The listing builds one solid part. Answer for the finished solid, in the listing's coordinates (mm). Round coordinates to 2 decimals unless told otherwise and drop trailing zeros. Loops run counter-clockwise (first coordinate to the right, second up) from the corner with the lowest first, then second, coordinate; pieces in that order, holes last. Notation, with made-up numbers: (32.5, 35) -> (76.5, 35) arc R21 cw to (76.5, 46) -> close; hole circle Ø3 at (66.5, 82.25). An arc over 180 degrees is marked (long way). One line per question, with ' | ' between items.
from build123d import *

# Parameters (mm, degrees)
BOSS_EXTRUDE1_DEPTH = 2
CUT_EXTRUDE4_START  = -2
CUT_EXTRUDE4_DEPTH  = 2


# Read off the part's stored shape, not the designer's step: Cut-Extrude4
with BuildPart() as part:
    # Sketch1 → Boss-Extrude1 (new body)
    with BuildSketch(Plane.XY):
        with BuildLine():
            Line((0, 76.134146341), (0, -0.865853659))
            ThreePointArc((0, -0.865853659), (-0.439339828, -1.92651383), (-1.5, -2.365853659))
            Line((-1.5, -2.365853659), (-5, -2.365853659))
            Line((-5, -2.365853659), (-5, 77.634146341))
            Line((-5, 77.634146341), (-1.5, 77.634146341))
            ThreePointArc((-1.5, 77.634146341), (-0.439339828, 77.194806513), (0, 76.134146341))
        make_face()
    extrude(amount=BOSS_EXTRUDE1_DEPTH)

    # Cut-Extrude4 outline → Cut-Extrude4 (cut)
    with BuildSketch(Plane.XY.offset(2).offset(CUT_EXTRUDE4_START)):
        Polygon((-5, 77.634146341), (-5, 75.884146341), (-3.25, 77.634146341), align=None)
        Polygon((-3.75, -2.365853659), (-5, -1.115853659), (-5, -2.365853659), align=None)
        Polygon((-3.25, 0.634146341), (-5, 2.384146341), (-5, -1.115853659), align=None)
        Polygon((-3.25, 4.134146341), (-5, 5.884146341), (-5, 2.384146341), align=None)
        Polygon((-3.25, 7.634146341), (-5, 9.384146341), (-5, 5.884146341), align=None)
        Polygon((-3.25, 11.134146341), (-5, 12.884146341), (-5, 9.384146341), align=None)
        Polygon((-3.25, 14.634146341), (-5, 16.384146341), (-5, 12.884146341), align=None)
        Polygon((-3.25, 18.134146341), (-5, 19.884146341), (-5, 16.384146341), align=None)
        Polygon((-3.25, 21.634146341), (-5, 23.384146341), (-5, 19.884146341), align=None)
        Polygon((-3.25, 25.134146341), (-5, 26.884146341), (-5, 23.384146341), align=None)
        Polygon((-3.25, 28.634146341), (-5, 30.384146341), (-5, 26.884146341), align=None)
        Polygon((-3.25, 32.134146341), (-5, 33.884146341), (-5, 30.384146341), align=None)
        Polygon((-3.25, 35.634146341), (-5, 37.384146341), (-5, 33.884146341), align=None)
        Polygon((-3.25, 39.134146341), (-5, 40.884146341), (-5, 37.384146341), align=None)
        Polygon((-3.25, 42.634146341), (-5, 44.384146341), (-5, 40.884146341), align=None)
        Polygon((-3.25, 46.134146341), (-5, 47.884146341), (-5, 44.384146341), align=None)
        Polygon((-3.25, 49.634146341), (-5, 51.384146341), (-5, 47.884146341), align=None)
        Polygon((-3.25, 53.134146341), (-5, 54.884146341), (-5, 51.384146341), align=None)
        Polygon((-3.25, 56.634146341), (-5, 58.384146341), (-5, 54.884146341), align=None)
        Polygon((-3.25, 60.134146341), (-5, 61.884146341), (-5, 58.384146341), align=None)
        Polygon((-3.25, 63.634146341), (-5, 65.384146341), (-5, 61.884146341), align=None)
        Polygon((-3.25, 67.134146341), (-5, 68.884146341), (-5, 65.384146341), align=None)
        Polygon((-3.25, 70.634146341), (-5, 72.384146341), (-5, 68.884146341), align=None)
        Polygon((-3.25, 74.134146341), (-5, 75.884146341), (-5, 72.384146341), align=None)
    extrude(amount=CUT_EXTRUDE4_DEPTH, mode=Mode.SUBTRACT)


solid = part.part
Q1. For a pull along Y with two mould halves and no side action, classify faces 1 (the face through (0, 38, 1)), 2 (the face through (-4.137, 13.747, 0.986)), 3 (the face through (-4.137, 20.747, 0.986)) as pulls with the +Y half, pulls with the -Y half, needs draft (parallel to the pull), parting line crosses it, or undercut.
Numbers:
face 1: needs draft | face 2: undercut | face 3: undercut
Q2. Find the intervals of material crossed by line 1 (Y direction, x = -1.35, z = 1.1); line 2 (Y direction, x = -0.4, z = 0.9); line 3 (X direction, y = 49, z = 1.2), in increasing order. Write a range as from..to.
Numbers:
line 1: -2.36..77.63 | line 2: -1.89..77.15 | line 3: -3.88..0
Q3. A cutting plane is placed at A-A on y = 12. Give the vertices of the cut face in (x, z).
Numbers:
outline: (-4.12, 0) -> (0, 0) -> (0, 2) -> (-4.12, 2) -> close
